```python
from build123d import *

# Parameters (mm, degrees)
SKETCH2_W           = 17.853706718
SKETCH2_H           = 10
BOSS_EXTRUDE2_DEPTH = 5
SKETCH4_W           = 7.1
SKETCH4_H           = 1.928064037
CUT_EXTRUDE1_DEPTH  = 9.3
CUT_EXTRUDE4_START  = 1.02
SKETCH6_W           = 15.11279267
SKETCH6_H           = 6.275441998
CUT_EXTRUDE4_DEPTH  = 9.3
SKETCH7_R           = 1.65
CUT_EXTRUDE7_DEPTH  = 17.583123952
SKETCH9_W           = 9.168085379
SKETCH9_H           = 5.824430712
CUT_EXTRUDE8_DEPTH  = 17.304612844


with BuildPart() as part:
    # Sketch2 → Boss-Extrude2 (new body)
    with BuildSketch(Plane(origin=(0, 0, 0), x_dir=(1, 0, 0), z_dir=(0, 1, 0))):
        with Locations((6.073146641, 0)):
            Rectangle(SKETCH2_W, SKETCH2_H)
    extrude(amount=BOSS_EXTRUDE2_DEPTH)

    # Sketch4 → Cut-Extrude1 (cut)
    with BuildSketch(Plane.ZY.offset(2.853706718)):
        with Locations((-0.07, 1.984032018)):
            Rectangle(SKETCH4_W, SKETCH4_H)
    extrude(amount=-CUT_EXTRUDE1_DEPTH, mode=Mode.SUBTRACT)

    # Sketch6 → Cut-Extrude4 (cut)
    with BuildSketch(Plane(origin=(0, 0, 0), x_dir=(1, 0, 0), z_dir=(0, 1, 0)).offset(CUT_EXTRUDE4_START)):
        Rectangle(SKETCH6_W, SKETCH6_H)
    extrude(amount=CUT_EXTRUDE4_DEPTH, mode=Mode.SUBTRACT)

    # Sketch7 → Cut-Extrude7 (cut, through all)
    with BuildSketch(Plane.XZ):
        with Locations(Location((11.326869327, 0.023099137, 0), (0, 0, 270))):
            Circle(SKETCH7_R)
    extrude(amount=-CUT_EXTRUDE7_DEPTH, mode=Mode.SUBTRACT)

    # Sketch9 → Cut-Extrude8 (cut, through all)
    with BuildSketch(Plane(origin=(0, 1.02, 0), x_dir=(1, 0, 0), z_dir=(0, 1, 0))):
        with Locations((2.693538698, 0.026964957)):
            Rectangle(SKETCH9_W, SKETCH9_H)
    extrude(amount=-CUT_EXTRUDE8_DEPTH, mode=Mode.SUBTRACT)


solid = part.part
```
Input: part model. Units: mm. Frame: model coordinates. A direction names the side the tool comes from. Give positions to 0.01 mm unless a question says otherwise; leave off trailing zeros. Order: outer loops, then holes, each group sorted by start corner. A loop starts at its lowest first (then second) coordinate and runs counter-clockwise, first axis right, second up. Notation, with made-up numbers: (84, 39) - (88, 39) arc R13 ccw to (88, 49) - close; hole circle Ø5 at (38, -17.75). An arc over 180 degrees is marked (long way). One line per item, written item: value.
1. Line query: probe 1 along Z at (x, y) = (-1.25, 0.9); probe 2 along Z at (x, y) = (5.25, 3.2); probe 3 along Y at (x, z) = (-0.5, 3). Output: solid intervals per line, ascending.
Determined:
probe 1: -5 to -2.94, 2.89 to 5
probe 2: -5 to -3.14, 3.14 to 5
probe 3: 0 to 1.02
2. Pin query (flat end, axial travel): pin 1 Ø5.5 at (x, z) = (1.5, -0.5) entering from +Y; pin 2 Ø1.5 at (y, z) = (4.5, -2) entering from -X. Return the tip coordinate at first contact, or that it passes through.
Determined:
pin 1: y = 5
pin 2: x = 7.56
3. Cut plane D-D, the plane y = 0.7. Output: boundary loops of the cut face in (x, z), and give its area (3 significant figures).
Determined:
outline: (-2.85, -5) - (15, -5) - (15, 5) - (-2.85, 5) - close; hole (-1.89, -2.94) - (7.28, -2.94) - (7.28, 2.89) - (-1.89, 2.89) - close; hole circle Ø3.3 at (11.33, 0.02)
area: 117 mm2
4. Cut plane A-A, the plane z = -2. Output: boundary loops of the cut face in (x, y).
Determined:
outline: (-2.85, 0) - (-1.89, 0) - (-1.89, 1.02) - (-2.85, 1.02) - close; (7.28, 0) - (15, 0) - (15, 5) - (7.56, 5) - (7.56, 1.02) - (7.28, 1.02) - close
5. Draft query along Z for faces 1 (the face through (6, 2, -5)), 2 (the face through (-2.854, 0.8, 0.1)), 3 (the face through (7.278, 0.5, 0)). Return one class per face: released by +Z, released by -Z, zero draft, split by the parting line, or undercut.
Determined:
face 1: released by -Z
face 2: zero draft
face 3: undercut
6. Reachability of faces 4 (the face through (2, 4, -3.138)), 5 (the face through (2, 2, 3.48)), 6 (the face through (2.6, 0.5, 2.885)) from +Z, -Z, +X, -X, +Y, -Y: full face, straight path, thin tool, end or side. Return the list, or none.
Determined:
face 4: -X, +Y
face 5: -X
face 6: +Y, -Y
7. Cut plane C-C, the plane y = 2.4. Output: boundary loops of the cut face in (x, z).
Determined:
outline: (-2.85, -5) - (15, -5) - (15, 5) - (-2.85, 5) - (-2.85, 3.48) - (6.45, 3.48) - (6.45, 3.14) - (7.56, 3.14) - (7.56, -3.14) - (6.45, -3.14) - (6.45, -3.62) - (-2.85, -3.62) - close; hole circle Ø3.3 at (11.33, 0.02)
8. Cut plane B-B, the plane x = 0.25. Output: boundary loops of the cut face in (y, z).
Determined:
outline: (0, -5) - (5, -5) - (5, -3.14) - (2.95, -3.14) - (2.95, -3.62) - (1.02, -3.62) - (1.02, -2.94) - (0, -2.94) - close; (0, 2.89) - (1.02, 2.89) - (1.02, 3.48) - (2.95, 3.48) - (2.95, 3.14) - (5, 3.14) - (5, 5) - (0, 5) - close
